```python
from build123d import *

# Parameters (mm, degrees)
F1_DEPTH = 35
F2_W     = 50
F2_H     = 26
F3_DEPTH = 20


with BuildPart() as f1:
    # F0 (on Front) → F1 (new body)
    with BuildSketch(Plane.XZ):
        Polygon((-50, 0), (0, 0), (0, 50), (-6, 50), (-50, 25), align=None)
    extrude(amount=F1_DEPTH)

    # F2 (on Front) → F3 (cut)
    with BuildSketch(Plane.XZ):
        with Locations((-25, 25)):
            Rectangle(F2_W, F2_H)
    extrude(amount=F3_DEPTH, mode=Mode.SUBTRACT)


solid = f1.part
```
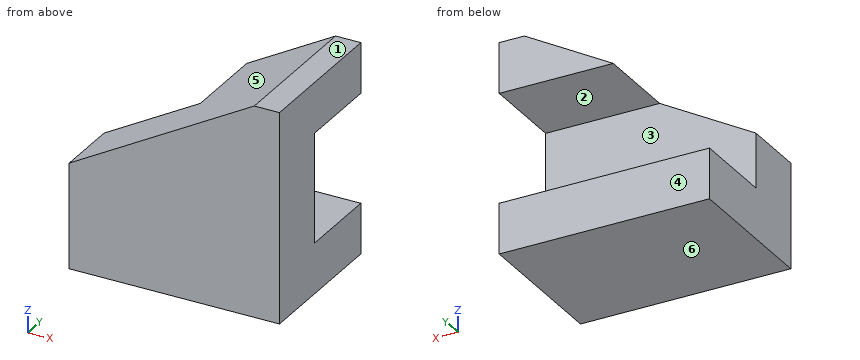
Model file for the job. Use its own axes, mm. Face numbers are marked on the shaded views. A direction names the side the tool comes from. Round coordinates to 2 decimals unless told otherwise and drop trailing zeros. Loops run counter-clockwise (first coordinate to the right, second up) from the corner with the lowest first, then second, coordinate; pieces in that order, holes last. Notation, with made-up numbers: M 59.5,0 L 100.5,0 A6 ccw 100.5,9 Z; hole C 38.5,23.5 d4. An arc over 180 degrees is marked long. Put each result on its own line as item: value. Start each with the question number.
Item 1: Cut at C-C (z = 26). List the corners of the cut face in (x, y), then the cut area to 3 significant figures.
Item 2: Mould opens along Z. For the marked faces 3, 4, 5 and 6 say: released by +Z, released by -Z, zero draft, split by the parting line, or undercut.
Item 3: Cut at A-A (y = -3). List the corners of the cut face in (x, z).
Item 4: Drill centre lines: line 1 along Z through (x, y) = (-3, -7.5); line 2 along Z through (x, y) = (-31.5, -14); line 3 along Z through (x, y) = (-18, -2.5). Where is each one in solid material? Low to high.
Item 5: Cut at D-D (x = -15.5). List the corners of the cut face in (y, z).
Item 6: 3-axis set-ups, long thin cutter, end or side, ignore diameter. For the marked faces 1 and 2: which of +Z, -Z, +X, -X, +Y, -Y reach the whole face in a straight line?
Item 7: Cut at B-B (y = -21). List the corners of the cut face in (x, z), then the cut area to 3 significant figures.
Item 8: Drop flat-ended pins along their axis: P1, Ø8, axis at x = -44.5, y = -17, coming from the +Z side; P2, Ø1.5, axis at x = -24.5, y = -4.5, coming from the +Z side; P3, Ø16, axis at x = -30, y = -12.5, coming from the +Z side. Give the stop position or say it passes through.
Answer block:
1. outline: M -48.24,-35 L 0,-35 L 0,-20 L -48.24,-20 Z
1. area: 724 mm2
2. face 3: undercut
2. face 4: zero draft
2. face 5: released by +Z
2. face 6: released by -Z
3. outline: M -50,0 L 0,0 L 0,12 L -50,12 Z; M -27.12,38 L 0,38 L 0,50 L -6,50 Z
4. line 1: 0 to 12, 38 to 50
4. line 2: 0 to 12
4. line 3: 0 to 12, 38 to 43.18
5. outline: M -35,0 L 0,0 L 0,12 L -20,12 L -20,38 L 0,38 L 0,44.6 L -35,44.6 Z
6. face 1: +Z, +X, -X, +Y, -Y
6. face 2: +X, -X, +Y
7. outline: M -50,0 L 0,0 L 0,50 L -6,50 L -50,25 Z
7. area: 1,950 mm2
8. P1: z = 29.63
8. P2: z = 39.91
8. P3: z = 40.91
